Can you work these out from the model? Positions are in its coordinate system, mm. Face numbers are marked on the shaded views. A direction names the side the tool comes from. Give positions to 0.01 mm unless a question says otherwise; leave off trailing zeros. Loops run counter-clockwise (first coordinate to the right, second up) from the corner with the lowest first, then second, coordinate; pieces in that order, holes last. Notation, with made-up numbers: (-26, 39.5) -> (23, 39.5) arc R22 cw to (23, 65.5) -> close; hole circle Ø5 at (-31.5, -9.75). An arc over 180 degrees is marked (long way). One line per question, with ' | ' between items.
from build123d import *

# Parameters (mm, degrees)
ESQUISSE2_R             = 5.196152423
BOSS_EXTRU_1_DEPTH      = 0.5
ESQUISSE3_R             = 2.5
BOSS_EXTRU_2_DEPTH      = 6
ESQUISSE4_R             = 2
BOSS_EXTRU_3_DEPTH      = 4
CHANFREIN1_SIZE         = 0.5
ENL_V_MAT_EXTRU_2_DEPTH = 2


with BuildPart() as part:
    # Esquisse1 → Base-Révolution (revolve)
    with BuildSketch(Plane.XY):
        with BuildLine():
            Line((0, 3), (5.196152423, 3))
            ThreePointArc((5.196152423, 3), (3, 5.196152423), (0, 6))
            Line((0, 6), (0, 3))
        make_face()
    revolve(axis=Axis((0, 0, 0), (0, 1, 0)))

    # Esquisse2 → Boss.-Extru.1 (add)
    with BuildSketch(Plane.XZ.offset(-3)):
        Circle(ESQUISSE2_R)
    extrude(amount=BOSS_EXTRU_1_DEPTH)

    # Esquisse3 → Boss.-Extru.2 (add)
    with BuildSketch(Plane.XZ.offset(-2.5)):
        Circle(ESQUISSE3_R)
    extrude(amount=BOSS_EXTRU_2_DEPTH)

    # Esquisse4 → Boss.-Extru.3 (add)
    with BuildSketch(Plane.XZ.offset(3.5)):
        Circle(ESQUISSE4_R)
    extrude(amount=BOSS_EXTRU_3_DEPTH)

    # Chanfrein1
    chanfrein1_edges = [part.edges().sort_by_distance(p)[0] for p in [
        (-2, -7.5, 0),
    ]]
    chamfer(chanfrein1_edges, length=CHANFREIN1_SIZE)

    # Esquisse5 → Enlèv. mat.-Extru.2 (cut)
    with BuildSketch(Plane.XZ.offset(-6.5)):
        with BuildLine():
            Line((-0.5, -2.5), (-0.5, -0.866025404))
            ThreePointArc((-0.5, -0.866025404), (-0.707106781, -0.707106781), (-0.866025404, -0.5))
            Line((-0.866025404, -0.5), (-2.5, -0.5))
            Line((-2.5, -0.5), (-2.5, 0.5))
            Line((-2.5, 0.5), (-0.866025404, 0.5))
            ThreePointArc((-0.866025404, 0.5), (-0.707106781, 0.707106781), (-0.5, 0.866025404))
            Line((-0.5, 0.866025404), (-0.5, 2.5))
            Line((-0.5, 2.5), (0.5, 2.5))
            Line((0.5, 2.5), (0.5, 0.866025404))
            ThreePointArc((0.5, 0.866025404), (0.707106781, 0.707106781), (0.866025404, 0.5))
            Line((0.866025404, 0.5), (2.5, 0.5))
            Line((2.5, 0.5), (2.5, -0.5))
            Line((2.5, -0.5), (0.866025404, -0.5))
            ThreePointArc((0.866025404, -0.5), (0.707106781, -0.707106781), (0.5, -0.866025404))
            Line((0.5, -0.866025404), (0.5, -2.5))
            Line((0.5, -2.5), (-0.5, -2.5))
        make_face()
    extrude(amount=ENL_V_MAT_EXTRU_2_DEPTH, mode=Mode.SUBTRACT)


solid = part.part
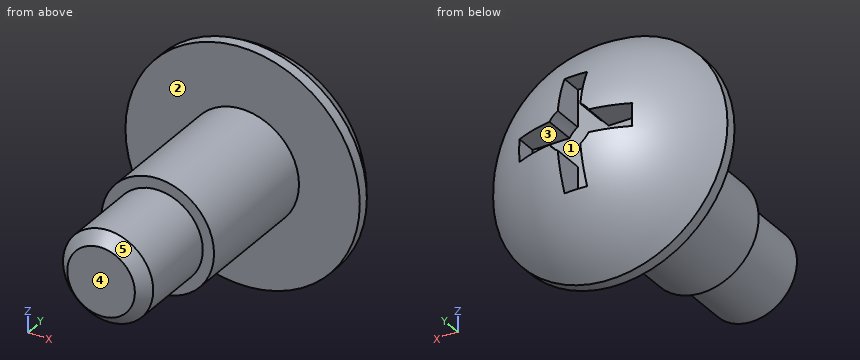
Q1. If we mould it in two halves opening along Z, with no side actions, what happens to the marked faces 3, 4 and 5? For each: pulls with the +Z half, pulls with the -Z half, needs draft (parallel to the pull), parting line crosses it, or undercut.
Entries:
face 3: undercut | face 4: needs draft | face 5: parting line crosses it
Q2. If we section it at C-C (z = 0): Write out the boundary of the cut face in (x, y), plus the area to 3 significant figures.
Entries:
outline: (-5.2, 2.5) -> (-2.5, 2.5) -> (-2.5, -3.5) -> (-2, -3.5) -> (-2, -7) -> (-1.5, -7.5) -> (1.5, -7.5) -> (2, -7) -> (2, -3.5) -> (2.5, -3.5) -> (2.5, 2.5) -> (5.2, 2.5) -> (5.2, 3) arc R6 ccw to (2.5, 5.45) -> (2.5, 4.5) -> (-2.5, 4.5) -> (-2.5, 5.45) arc R6 ccw to (-5.2, 3) -> close | area: 66.4 mm²
Q3. On a 3-axis mill with a long thin cutter (end or side, diameter ignored), from which of +Z, -Z, +X, -X, +Y, -Y can I reach the whole of each face in a straight line? I mean the marked faces 1 and 2. Say none if no direction works.
Entries:
face 1: +Y | face 2: -Y
Q4. If I drill on probe 1 along Z at (x, y) = (-1.5, 1.5); probe 2 along Y at (x, z) = (-0.25, 0.75), over which ranges is the centre line in solid material (lowest first)? Write a range as from..to.
Entries:
probe 1: -2..2 | probe 2: -7.5..4.5
Q5. If we section it at A-A (x = 0): Write out the boundary of the cut face in (y, z).
Entries:
outline: (-7.5, -1.5) -> (-7, -2) -> (-3.5, -2) -> (-3.5, -2.5) -> (2.5, -2.5) -> (2.5, -5.2) -> (3, -5.2) arc R6 ccw to (5.45, -2.5) -> (4.5, -2.5) -> (4.5, 2.5) -> (5.45, 2.5) arc R6 ccw to (3, 5.2) -> (2.5, 5.2) -> (2.5, 2.5) -> (-3.5, 2.5) -> (-3.5, 2) -> (-7, 2) -> (-7.5, 1.5) -> close
Q6. For pin 1 Ø1.6 at (y, z) = (5, 1.5) entering from -X; pin 2 Ø3 at (x, y) = (4, 4) entering from +Z; pin 3 Ø0.5 at (y, z) = (5, 0) entering from -X, each with a flat end and sliding along its axis, tell me the tip position at first contact or that it passes through.
Entries:
pin 1: x = -4.06 | pin 2: z = 4.32 | pin 3: x = -3.67
Q7. If we section it at B-B (y = 5.25): Write out the boundary of the cut face in (x, z).
Entries:
outline: circle Ø5.81 at (0, 0); hole (-2.5, -0.5) -> (-0.87, -0.5) arc R1 ccw to (-0.5, -0.87) -> (-0.5, -2.5) -> (0.5, -2.5) -> (0.5, -0.87) arc R1 ccw to (0.87, -0.5) -> (2.5, -0.5) -> (2.5, 0.5) -> (0.87, 0.5) arc R1 ccw to (0.5, 0.87) -> (0.5, 2.5) -> (-0.5, 2.5) -> (-0.5, 0.87) arc R1 ccw to (-0.87, 0.5) -> (-2.5, 0.5) -> close
Q8. If we section it at D-D (y = 2): Write out the boundary of the cut face in (x, z).
Entries:
outline: circle Ø5 at (0, 0)
